CAD build for the part. Positions are in the model's coordinates, mm. Face numbers are marked on the shaded views. A direction names the side the tool comes from. Coordinates: 2 decimals unless noted, no trailing zeros. Loops run counter-clockwise (first coordinate to the right, second up) from the corner with the lowest first, then second, coordinate; pieces in that order, holes last.
1) Which spindle directions (+Z, -Z, +X, -X, +Y, -Y) get a long thin tool onto all of the face, cutting with end or side? Do the marked faces 5, 6, 7 and 8. Say none if no direction does.
2) Saw through at B-B, the plane x = 0. Write the cut outline in (y, z).
3) Saw through at A-A, the plane z = -6.5. Write the cut outline in (x, y).
4) Pin check, flat tips, straight feed: pin 1 Ø1.5 at (x, z) = (3, -2) entering from -Y; pin 2 Ø5.5 at (x, y) = (-30, 0) entering from -Z; pin 3 Ø5 at (x, z) = (4.5, -4) entering from +Y. Stop position of each tip, or through.
5) Saw through at D-D, the plane x = 11. Write the cut outline in (y, z).
6) Saw through at C-C, the plane y = -23.72. Write the cut outline in (x, z).
7) Two-plate mould, pull along Y, no slides. Class the marked faces 1, 2, 3 and 4: +Y half, -Y half, draft (parallel to the pull), parting line (faces both ways), or undercut.
8) Wall check: line 1 along X through (y, z) = (-9.3, -3.25); line 2 along X through (y, z) = (13, -4.5); line 3 along Y through (x, z) = (12, -5.75). Give the ranges that are in metal, low to high.
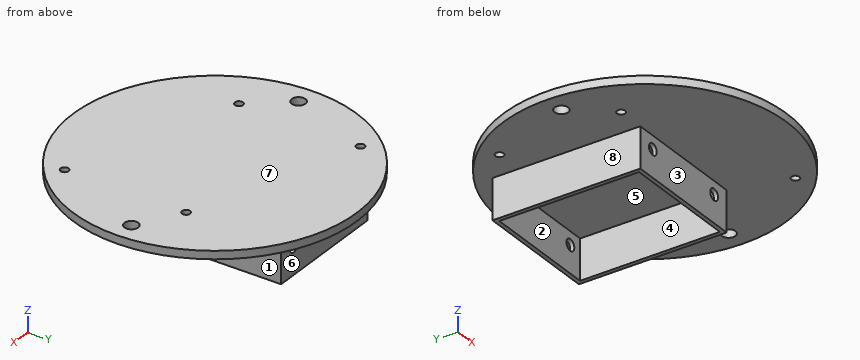
```python
from build123d import *

# Parameters (mm, degrees)
SKETCH1_R                      = 35
BOSS_EXTRUDE1_DEPTH            = 2
SKETCH2_W                      = 31
SKETCH2_H                      = 36.5
SKETCH2_W_2                    = 29
SKETCH2_H_2                    = 34.5
BOSS_EXTRUDE2_DEPTH            = 10
SKETCH3_R                      = 1
CUT_EXTRUDE1_DEPTH             = 10
CUT_EXTRUDE2_REACH             = 58.721
SKETCH5_R                      = 1.4
CUT_EXTRUDE2_DIRECTION_2_REACH = 58.721
SKETCH6_R                      = 1.7
CUT_EXTRUDE3_DEPTH             = 51.931326313


with BuildPart() as part:
    # Sketch1 → Boss-Extrude1 (new body)
    with BuildSketch(Plane.XY):
        Circle(SKETCH1_R)
    extrude(amount=BOSS_EXTRUDE1_DEPTH)

    # Sketch2 → Boss-Extrude2 (add)
    with BuildSketch(Plane(origin=(0, 0, 0), x_dir=(-1, 0, 0), z_dir=(0, 0, -1))):
        with Locations((0, 8.75)):
            Rectangle(SKETCH2_W, SKETCH2_H)
        with Locations((0, 8.75)):
            Rectangle(SKETCH2_W_2, SKETCH2_H_2, mode=Mode.SUBTRACT)
    extrude(amount=BOSS_EXTRUDE2_DEPTH)

    # Sketch3 → Cut-Extrude1 (cut)
    with BuildSketch(Plane(origin=(0, 0, 0), x_dir=(-1, 0, 0), z_dir=(0, 0, -1))):
        with Locations((22.366777203, 20.53)):
            Circle(SKETCH3_R)
        with Locations((22.37, -9.469999827)):
            Circle(SKETCH3_R)
        with Locations((-19.48, 6.28)):
            Circle(SKETCH3_R)
        with Locations((-19.48, -23.72)):
            Circle(SKETCH3_R)
    extrude(amount=-CUT_EXTRUDE1_DEPTH, mode=Mode.SUBTRACT)

    # Cut-Extrude2: up to this face of the body (flat: up to its plane)
    cut_extrude2_end = Plane(part.part.faces().sort_by_distance((0, -9.5, -5))[0])
    # Sketch5 → Cut-Extrude2 (cut, up to the picked face)
    with BuildSketch(Plane(origin=(0, -8.5, 0), x_dir=(1, 0, 0), z_dir=(0, 1, 0)), mode=Mode.PRIVATE) as cut_extrude2_sk1:
        with Locations((-11, 3.25)):
            Circle(SKETCH5_R)
    cut_extrude2_tool1 = split(extrude(cut_extrude2_sk1.sketch, amount=-CUT_EXTRUDE2_REACH, mode=Mode.PRIVATE), bisect_by=cut_extrude2_end, keep=Keep.BOTH, mode=Mode.PRIVATE)
    # Sketch5 → Cut-Extrude2 (cut, up to the picked face)
    with BuildSketch(Plane(origin=(0, -8.5, 0), x_dir=(1, 0, 0), z_dir=(0, 1, 0)), mode=Mode.PRIVATE) as cut_extrude2_sk2:
        with Locations((11, 3.25)):
            Circle(SKETCH5_R)
    cut_extrude2_tool2 = split(extrude(cut_extrude2_sk2.sketch, amount=-CUT_EXTRUDE2_REACH, mode=Mode.PRIVATE), bisect_by=cut_extrude2_end, keep=Keep.BOTH, mode=Mode.PRIVATE)
    add(cut_extrude2_tool1.solids().sort_by(Axis((-11, -8.5, -3.25), (0, -1, 0)))[0], mode=Mode.SUBTRACT)
    add(cut_extrude2_tool2.solids().sort_by(Axis((11, -8.5, -3.25), (0, -1, 0)))[0], mode=Mode.SUBTRACT)

    # Cut-Extrude2 direction 2: up to this face of the body (flat: up to its plane)
    cut_extrude2_direction_2_end = Plane(part.part.faces().sort_by_distance((0, 27, -5))[0])
    # Sketch5 → Cut-Extrude2 direction 2 (cut, up to the picked face)
    with BuildSketch(Plane(origin=(0, -8.5, 0), x_dir=(1, 0, 0), z_dir=(0, 1, 0)), mode=Mode.PRIVATE) as cut_extrude2_direction_2_sk1:
        with Locations((-11, 3.25)):
            Circle(SKETCH5_R)
    cut_extrude2_direction_2_tool1 = split(extrude(cut_extrude2_direction_2_sk1.sketch, amount=CUT_EXTRUDE2_DIRECTION_2_REACH, mode=Mode.PRIVATE), bisect_by=cut_extrude2_direction_2_end, keep=Keep.BOTH, mode=Mode.PRIVATE)
    # Sketch5 → Cut-Extrude2 direction 2 (cut, up to the picked face)
    with BuildSketch(Plane(origin=(0, -8.5, 0), x_dir=(1, 0, 0), z_dir=(0, 1, 0)), mode=Mode.PRIVATE) as cut_extrude2_direction_2_sk2:
        with Locations((11, 3.25)):
            Circle(SKETCH5_R)
    cut_extrude2_direction_2_tool2 = split(extrude(cut_extrude2_direction_2_sk2.sketch, amount=CUT_EXTRUDE2_DIRECTION_2_REACH, mode=Mode.PRIVATE), bisect_by=cut_extrude2_direction_2_end, keep=Keep.BOTH, mode=Mode.PRIVATE)
    add(cut_extrude2_direction_2_tool1.solids().sort_by(Axis((-11, -8.5, -3.25), (0, 1, 0)))[0], mode=Mode.SUBTRACT)
    add(cut_extrude2_direction_2_tool2.solids().sort_by(Axis((11, -8.5, -3.25), (0, 1, 0)))[0], mode=Mode.SUBTRACT)

    # Sketch6 → Cut-Extrude3 (cut, through all)
    with BuildSketch(Plane.XY.offset(2)):
        with Locations((30, 0)):
            Circle(SKETCH6_R)
        with Locations((-30, 0)):
            Circle(SKETCH6_R)
    extrude(amount=-CUT_EXTRUDE3_DEPTH, mode=Mode.SUBTRACT)


solid = part.part
```
Data:
1. face 5: -Z
1. face 6: -Z, +X, -X, +Y
1. face 7: +Z, +X, -X, +Y, -Y
1. face 8: -Z, -X, +Y, -Y
2. outline: (-35, 0) - (-9.5, 0) - (-9.5, -10) - (-8.5, -10) - (-8.5, 0) - (26, 0) - (26, -10) - (27, -10) - (27, 0) - (35, 0) - (35, 2) - (-35, 2) - close
3. outline: (-15.5, -9.5) - (15.5, -9.5) - (15.5, 27) - (-15.5, 27) - close; hole (-14.5, -8.5) - (14.5, -8.5) - (14.5, 26) - (-14.5, 26) - close
4. pin 1: stops at y = -9.5
4. pin 2: stops at z = 0
4. pin 3: stops at y = 27
5. outline: (-33.23, 0) - (-9.5, 0) - (-9.5, -1.85) - (-8.5, -1.85) - (-8.5, 0) - (26, 0) - (26, -1.85) - (27, -1.85) - (27, 0) - (33.23, 0) - (33.23, 2) - (-33.23, 2) - close; (-9.5, -10) - (-8.5, -10) - (-8.5, -4.65) - (-9.5, -4.65) - close; (26, -10) - (27, -10) - (27, -4.65) - (26, -4.65) - close
6. outline: (-25.74, 0) - (18.48, 0) - (18.48, 2) - (-25.74, 2) - close; (20.48, 0) - (25.74, 0) - (25.74, 2) - (20.48, 2) - close
7. face 1: draft
7. face 2: undercut
7. face 3: -Y half
7. face 4: undercut
8. line 1: x = -15.5 to -12.4, -9.6 to 9.6, 12.4 to 15.5
8. line 2: x = -15.5 to -14.5, 14.5 to 15.5
8. line 3: y = -9.5 to -8.5, 26 to 27
